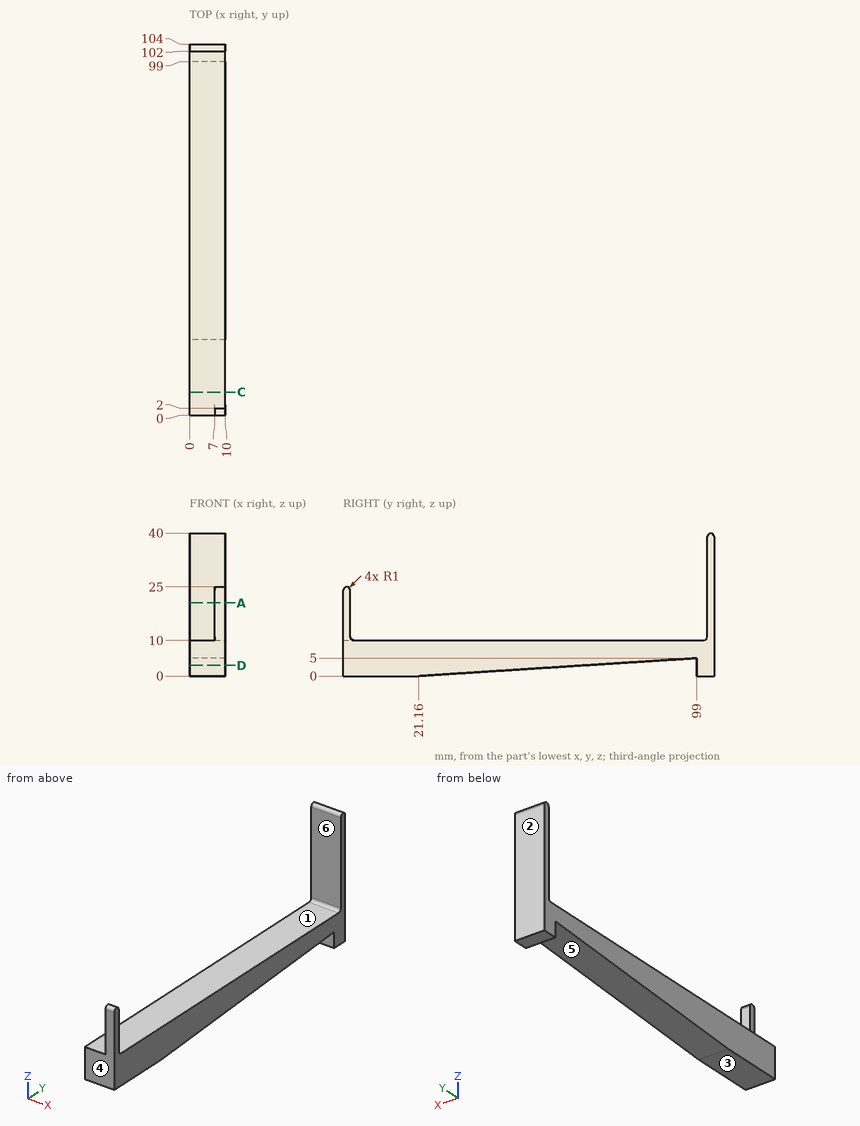
Here's the drawing with two shaded views (mm, measured from the low corner). I have some questions. A direction names the side the tool comes from. Round coordinates to 2 decimals unless told otherwise and drop trailing zeros. Order: outer loops, then holes, each group sorted by start corner. A loop starts at its lowest first (then second) coordinate and runs counter-clockwise, first axis right, second up. Notation, with made-up numbers: (75.25, -1.5) -> (104.25, -1.5) arc R9 cw to (104.25, 11.5) -> close; hole circle Ø9 at (12.5, 38.25). An arc over 180 degrees is marked (long way). Write each question's results on one line, items separated by ' | '. Start each with the question number.
Item 1: Thinking about a two-plate mould opening in Y: for the marked faces 1, 2 and 3, which applies, +Y half, -Y half, draft (parallel to the pull), parting line (faces both ways), or undercut?
Item 2: If we section it at A-A, the plane z = 20.5: Write out the boundary of the cut face in (x, y).
Item 3: Which directions (+Z, -Z, +X, -X, +Y, -Y) give clear straight access to the entire face, cutting with the end or side of a thin tool? Please do the marked faces 4, 5 and 6.
Item 4: Will these pins go through, and if not, where does the flat tip stop? pin 1 (1.5 mm diameter, centred on x = 3.5, z = 35, fed in from -Y); pin 2 (1.5 mm diameter, centred on x = 8.5, y = 90, fed in from +Z); pin 3 (0.9 mm diameter, centred on y = 2, z = 19, fed in from -X).
Item 5: If we section it at D-D, the plane z = 3: Write out the boundary of the cut face in (x, y) (1 decimal).
Item 6: Please list where these lines run through material, in increasing order: L1, parallel to Y at x = 8.75, z = 23; L2, parallel to Z at x = 0.5, y = 17.5; L3, parallel to Y at x = 2.75, z = 32.5.
Item 7: If we section it at C-C, the plane y = 6.5: Write out the boundary of the cut face in (x, z).
Results:
1) face 1: undercut | face 2: +Y half | face 3: draft
2) outline: (0, 102) -> (10, 102) -> (10, 104) -> (0, 104) -> close; (7, 0) -> (10, 0) -> (10, 2) -> (7, 2) -> close
3) face 4: +Z, -Z, +X, -X, -Y | face 5: -Z, +X, -X | face 6: +Z, +X, -X
4) pin 1: stops at y = 102 | pin 2: stops at z = 10 | pin 3: stops at x = 7
5) outline: (0, 0) -> (10, 0) -> (10, 67.9) -> (0, 67.9) -> close; (0, 99) -> (10, 99) -> (10, 104) -> (0, 104) -> close
6) L1: y = 0 to 2, 102 to 104 | L2: z = 0 to 10 | L3: y = 102 to 104
7) outline: (0, 0) -> (10, 0) -> (10, 10) -> (0, 10) -> close
